Source: CAD feature listing. Evaluate the final solid. Frame: model axes, mm. Face numbers are marked on the shaded views. A direction names the side the tool comes from. Give positions to 0.01 mm unless a question says otherwise; leave off trailing zeros. Write each loop counter-clockwise with the first axis right and the second up, starting at its lowest first coordinate (ties: lowest second). Pieces come first, ordered by that corner, then holes.
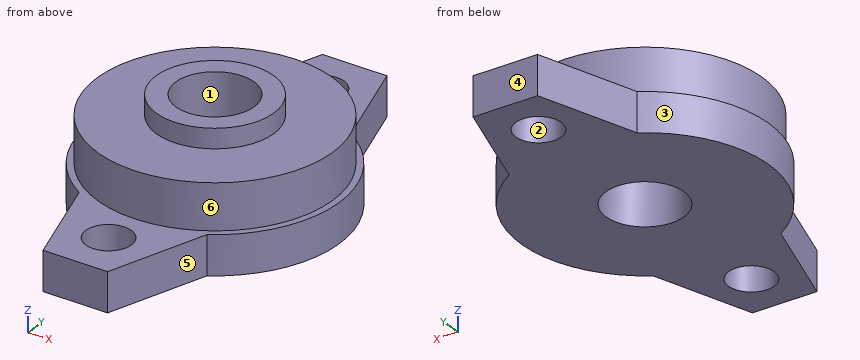
```python
from build123d import *

# Parameters (mm, degrees)
SKETCH_1_R          = 3.5
SKETCH_1_R_2        = 6
EXTRUDE_1_DEPTH     = 6
SKETCH_2_R          = 18
EXTRUDE_2_DEPTH     = 7
SKETCH_3_R          = 9
EXTRUDE_3_DEPTH     = 3
SKETCH_4_R          = 6
CUT_EXTRUDE_1_DEPTH = 41.115458367


with BuildPart() as part:
    # 草圖1 → 填料-伸長1 (new body)
    with BuildSketch(Plane.XY):
        with BuildLine():
            Line((-5, 31.5), (5, 31.5))
            Line((5, 31.5), (9.888283839, 16.224113002))
            ThreePointArc((9.888283839, 16.224113002), (19, 0), (9.888283839, -16.224113002))
            Line((9.888283839, -16.224113002), (5, -31.5))
            Line((5, -31.5), (-5, -31.5))
            Line((-5, -31.5), (-9.888283839, -16.224113002))
            ThreePointArc((-9.888283839, -16.224113002), (-19, 0), (-9.888283839, 16.224113002))
            Line((-9.888283839, 16.224113002), (-5, 31.5))
        make_face()
        with Locations((0, 24)):
            Circle(SKETCH_1_R, mode=Mode.SUBTRACT)
        with Locations((0, -24)):
            Circle(SKETCH_1_R, mode=Mode.SUBTRACT)
        Circle(SKETCH_1_R_2, mode=Mode.SUBTRACT)
    extrude(amount=EXTRUDE_1_DEPTH)

    # 草圖2 → 填料-伸長2 (add)
    with BuildSketch(Plane.XY.offset(6)):
        Circle(SKETCH_2_R)
    extrude(amount=EXTRUDE_2_DEPTH)

    # 草圖3 → 填料-伸長3 (add)
    with BuildSketch(Plane.XY.offset(13)):
        Circle(SKETCH_3_R)
    extrude(amount=EXTRUDE_3_DEPTH)

    # 草圖4 → 除料-伸長1 (cut, through all)
    with BuildSketch(Plane.XY.offset(16)):
        Circle(SKETCH_4_R)
    extrude(amount=-CUT_EXTRUDE_1_DEPTH, mode=Mode.SUBTRACT)


solid = part.part
```
1. Section query A-A (y = 0). Return loops of the section in (x, z).
2. Access query for the marked faces 5 and 6. Directions: +Z, -Z, +X, -X, +Y, -Y. A direction counts if a zero-diameter tool reaches every point of the face in a straight line with its end or side. Return the directions, or none.
3. Pin query (flat end, axial travel): P1, Ø9, axis at x = 0, y = -24, coming from the +Z side; P2, Ø4, axis at x = 6, y = 13, coming from the +Z side; P3, Ø5, axis at x = -14.5, z = 13.5, coming from the +Y side. Return the tip coordinate at first contact, or that it passes through.
4. Section query B-B (z = 3). Return loops of the section in (x, y), plus the area to 3 significant figures.
5. Pull-direction query (Y, two-part tool) for the marked faces 1, 2, 3 and 4; classes: pulls with the +Y half, pulls with the -Y half, needs draft (parallel to the pull), parting line crosses it, or undercut.
6. Line query: probe 1 along Y at (x, z) = (0, 4.3); probe 2 along Y at (x, z) = (0, 11.75); probe 3 along Z at (x, y) = (9, -11). Output: solid intervals per line, ascending.
7. Section query D-D (y = 24). Return loops of the section in (x, z), plus the area to 3 significant figures.
8. Section query C-C (x = 0). Return loops of the section in (y, z).
The answers:
1. outline: (-19, 0) - (-6, 0) - (-6, 16) - (-9, 16) - (-9, 13) - (-18, 13) - (-18, 6) - (-19, 6) - close; (6, 0) - (19, 0) - (19, 6) - (18, 6) - (18, 13) - (9, 13) - (9, 16) - (6, 16) - close
2. face 5: +Z, -Z, +X, -Y
2. face 6: +Z
3. P1: stops at z = 6
3. P2: stops at z = 13
3. P3: stops at y = 13.37
4. outline: (-9.89, -16.22) - (-5, -31.5) - (5, -31.5) - (9.89, -16.22) arc R19 ccw to (9.89, 16.22) - (5, 31.5) - (-5, 31.5) - (-9.89, 16.22) arc R19 ccw to start; hole circle Ø12 at (0, 0); hole circle Ø7 at (0, -24); hole circle Ø7 at (0, 24)
4. area: 1,320 mm2
5. face 1: undercut
5. face 2: undercut
5. face 3: parting line crosses it
5. face 4: pulls with the +Y half
6. probe 1: y = -31.5 to -27.5, -20.5 to -6, 6 to 20.5, 27.5 to 31.5
6. probe 2: y = -18 to -6, 6 to 18
6. probe 3: z = 0 to 13
7. outline: (-7.4, 0) - (-3.5, 0) - (-3.5, 6) - (-7.4, 6) - close; (3.5, 0) - (7.4, 0) - (7.4, 6) - (3.5, 6) - close
7. area: 46.8 mm2
8. outline: (-31.5, 0) - (-27.5, 0) - (-27.5, 6) - (-31.5, 6) - close; (-20.5, 0) - (-6, 0) - (-6, 16) - (-9, 16) - (-9, 13) - (-18, 13) - (-18, 6) - (-20.5, 6) - close; (6, 0) - (20.5, 0) - (20.5, 6) - (18, 6) - (18, 13) - (9, 13) - (9, 16) - (6, 16) - close; (27.5, 0) - (31.5, 0) - (31.5, 6) - (27.5, 6) - close
